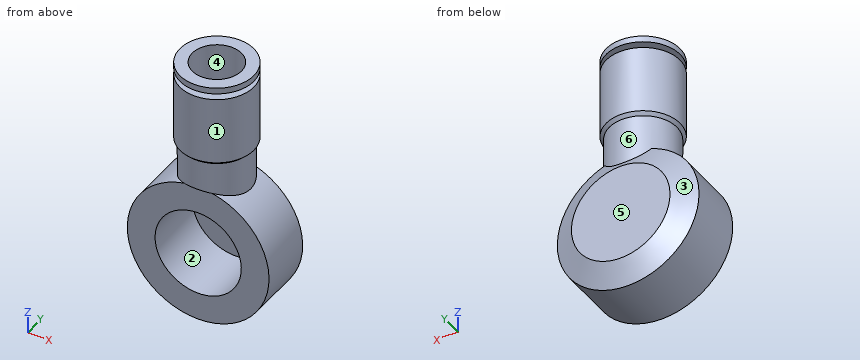
```python
from build123d import *

# Parameters (mm, degrees)
SKETCH2_R           = 5.5
BOSS_EXTRUDE4_DEPTH = 30
CUT_EXTRUDE1_START  = -2
SKETCH3_R           = 5.5
SKETCH3_R_2         = 4.5
CUT_EXTRUDE1_DEPTH  = 1
SKETCH5_R           = 11.5
CUT_EXTRUDE3_DEPTH  = 6
SKETCH8_R           = 4
CUT_EXTRUDE4_DEPTH  = 34
CUT_EXTRUDE6_START  = -1
SKETCH9_R           = 7
CUT_EXTRUDE6_DEPTH  = 34
BOSS_EXTRUDE5_START = -1
SKETCH10_R          = 6
SKETCH10_R_2        = 5.5
BOSS_EXTRUDE5_DEPTH = 1
BOSS_EXTRUDE6_START = -12
SKETCH11_R          = 6
SKETCH11_R_2        = 5.5
BOSS_EXTRUDE6_DEPTH = 12
CHAMFER1_SIZE       = 1


with BuildPart() as part:
    # Sketch1 → Revolve2 (revolve)
    with BuildSketch(Plane.XY, mode=Mode.PRIVATE) as revolve2_sk:
        Polygon((11.5, 3.5), (8, 5.5), (0, 5.5), (0, -5.5), (11.5, -5.5), align=None)
    revolve(revolve2_sk.sketch.rotate(Axis((0, 5.5, 0), (0, -1, 0)), 90), axis=Axis((0, 5.5, 0), (0, -1, 0)))

    # Sketch2 → Boss-Extrude4 (add)
    with BuildSketch(Plane.XY):
        with Locations(Location((0, -0.5, 0), (0, 0, 133.341758512))):
            Circle(SKETCH2_R)
    extrude(amount=BOSS_EXTRUDE4_DEPTH)

    # Sketch3 → Cut-Extrude1 (cut)
    with BuildSketch(Plane.XY.offset(30).offset(CUT_EXTRUDE1_START)):
        with Locations(Location((0, -0.5, 0), (0, 0, 133.341758512))):
            Circle(SKETCH3_R)
        with Locations((0, -0.5)):
            Circle(SKETCH3_R_2, mode=Mode.SUBTRACT)
    extrude(amount=CUT_EXTRUDE1_DEPTH, mode=Mode.SUBTRACT)

    # Sketch5 → Cut-Extrude3 (cut)
    with BuildSketch(Plane.XZ.offset(5.5)):
        Circle(SKETCH5_R)
    extrude(amount=CUT_EXTRUDE3_DEPTH, mode=Mode.SUBTRACT)

    # Sketch8 → Cut-Extrude4 (cut)
    with BuildSketch(Plane.XY.offset(30)):
        with Locations((0, -0.5)):
            Circle(SKETCH8_R)
    extrude(amount=-CUT_EXTRUDE4_DEPTH, mode=Mode.SUBTRACT)

    # Sketch9 → Cut-Extrude6 (cut)
    with BuildSketch(Plane(origin=(0, 5.5, 0), x_dir=(1, 0, 0), z_dir=(0, 1, 0)).offset(CUT_EXTRUDE6_START)):
        with Locations(Location((0, 0, 0), (0, 0, 270))):
            Circle(SKETCH9_R)
    extrude(amount=-CUT_EXTRUDE6_DEPTH, mode=Mode.SUBTRACT)

    # Sketch10 → Boss-Extrude5 (add)
    with BuildSketch(Plane.XY.offset(30).offset(BOSS_EXTRUDE5_START)):
        with Locations((0, -0.5)):
            Circle(SKETCH10_R)
        with Locations(Location((0, -0.5, 0), (0, 0, 133.341758512))):
            Circle(SKETCH10_R_2, mode=Mode.SUBTRACT)
    extrude(amount=BOSS_EXTRUDE5_DEPTH)

    # Sketch11 → Boss-Extrude6 (add)
    with BuildSketch(Plane.XY.offset(28).offset(BOSS_EXTRUDE6_START)):
        with Locations((0, -0.5)):
            Circle(SKETCH11_R)
        with Locations(Location((0, -0.5, 0), (0, 0, 133.341758512))):
            Circle(SKETCH11_R_2, mode=Mode.SUBTRACT)
    extrude(amount=BOSS_EXTRUDE6_DEPTH)

    # Chamfer1
    # the kernel refuses this chamfer: 1 mm, written as the material it takes off along each edge
    with BuildSketch(Plane(origin=(0, -0.5, 16), x_dir=(1, 0, 0), z_dir=(0, -1, 0))) as chamfer1_piece_1_section:
        Polygon((6 - CHAMFER1_SIZE, 0), (6, CHAMFER1_SIZE), (6, 0), align=None)
    chamfer1_piece_1 = revolve(axis=Axis((0, -0.5, 16), (0, 0, 1)), mode=Mode.PRIVATE)
    chamfer1_piece_1 = chamfer1_piece_1 - Plane(origin=(0, -0.5, 16.746748463), x_dir=(-0.6863485886393825, 0.7272727238613639, 0), z_dir=(0, 0, -1)) * Cylinder(5.5, 25, mode=Mode.PRIVATE)
    add(chamfer1_piece_1, mode=Mode.SUBTRACT)


solid = part.part
```
Build history of the part. All positions in model axes, mm. Face numbers are marked on the shaded views. A direction names the side the tool comes from. Coordinates: 2 decimals unless noted, no trailing zeros. Order: outer loops, then holes, each group sorted by start corner. A loop starts at its lowest first (then second) coordinate and runs counter-clockwise, first axis right, second up.
Item 1: Saw through at B-B on z = 0. List the corners of the cut face in (x, y).
Filled in:
outline: (-11.5, -5.5) - (-7, -5.5) - (-7, 4.5) - (7, 4.5) - (7, -5.5) - (11.5, -5.5) - (11.5, 3.5) - (8, 5.5) - (-8, 5.5) - (-11.5, 3.5) - close
Item 2: Mould opens along X. For the marked faces 4, 5 and 6 say: released by +X, released by -X, zero draft, split by the parting line, or undercut.
Filled in:
face 4: undercut
face 5: zero draft
face 6: split by the parting line
Item 3: Drop flat-ended pins along their axis: pin 1 Ø8 at (x, z) = (5.5, 21) entering from -Y; pin 2 Ø2 at (y, z) = (4, 19) entering from +X; pin 3 Ø3 at (y, z) = (3, 18.5) entering from +X. Give the stop position or say it passes through.
Filled in:
pin 1: stops at y = -6.31
pin 2: stops at x = 4.87
pin 3: stops at x = 5.66
Item 4: Saw through at C-C on y = -0.5. List the corners of the cut face in (x, z), then the cut area to 3 significant figures.
Filled in:
outline: (-6, 17) - (-5.5, 16.5) - (-5.5, 10.1) arc R11.5 ccw (long way) to (5.5, 10.1) - (5.5, 16.5) - (6, 17) - (6, 28) - (4.5, 28) - (4.5, 29) - (6, 29) - (6, 30) - (4, 30) - (4, 5.74) arc R7 cw (long way) to (-4, 5.74) - (-4, 30) - (-6, 30) - (-6, 29) - (-4.5, 29) - (-4.5, 28) - (-6, 28) - close
area: 293 mm2
Item 5: Saw through at D-D on z = 26. List the corners of the cut face in (x, y), then the cut area to 3 significant figures.
Filled in:
outline: circle Ø12 at (0, -0.5); hole circle Ø8 at (0, -0.5)
area: 62.8 mm2
Item 6: Tool access for the marked faces 1, 2 and 3: list every direction of +Z, -Z, +X, -X, +Y, -Y with a clear straight run to the whole face (end or side of a thin tool).
Filled in:
face 1: +Z
face 2: -Y
face 3: +Y
Item 7: Drill centre lines: L1, parallel to X at y = 1.25, z = 0; L2, parallel to X at y = -0.5, z = 15.75; L3, parallel to Y at x = 0, z = 23. Where is each one in solid material? Low to high.
Filled in:
L1: x = -11.5 to -7, 7 to 11.5
L2: x = -5.5 to -4, 4 to 5.5
L3: y = -6.5 to -4.5, 3.5 to 5.5
